The listing builds one solid part. Answer for the finished solid, in the listing's coordinates (mm). Coordinates: 2 decimals unless noted, no trailing zeros. Loops run counter-clockwise (first coordinate to the right, second up) from the corner with the lowest first, then second, coordinate; pieces in that order, holes last. Notation, with made-up numbers: M -5.5,-21.75 L 37.5,-21.75 A14 cw 37.5,-7.75 Z; hole C -14,26 d3. An arc over 180 degrees is marked long. Answer in a Markdown table with one row per item. Add a question column.
from build123d import *

# Parameters (mm, degrees)
SKETCH2_W           = 40
SKETCH2_H           = 80
BOSS_EXTRUDE1_DEPTH = 5
CUT_EXTRUDE1_DEPTH  = 2.8000000000000003
CUT_EXTRUDE2_DEPTH  = 1
CUT_EXTRUDE3_DEPTH  = 1
CUT_EXTRUDE4_DEPTH  = 0.5
CUT_EXTRUDE5_DEPTH  = 0.5
FILLET1_R           = 0.5
FILLET2_R           = 2.5
F_3DSKETCH6_R       = 1.5500000000000003
F_3DSKETCH6_R_2     = 0.8500000000000008
CUT_EXTRUDE6_DEPTH  = 2.1
FILLET3_START       = -10.446006344
FILLET3_DEPTH       = 8.020486493
FILLET3_START_2     = 2.417038032
FILLET3_2_DEPTH     = 8.020486493


with BuildPart() as part:
    # Sketch2 → Boss-Extrude1 (new body)
    with BuildSketch(Plane(origin=(0, 0, 0), x_dir=(1, 0, 0), z_dir=(0, 1, 0))):
        Rectangle(SKETCH2_W, SKETCH2_H)
    extrude(amount=BOSS_EXTRUDE1_DEPTH)

    # 3DSketch1 → Cut-Extrude1 (cut)
    with BuildSketch(Plane(origin=(-16.51128006150057, 0, -37.5), x_dir=(0.4458957716594368, 0, 0.8950848902848463), z_dir=(0, 1, 0))):
        Polygon((0, 0), (14.72461992821574, 29.557994604621218), (74.05892188684597, 0), (59.334301958630235, -29.557994604621218), align=None)
    extrude(amount=CUT_EXTRUDE1_DEPTH, mode=Mode.SUBTRACT)

    # 3DSketch2 → Cut-Extrude2 (cut)
    with BuildSketch(Plane(origin=(2.4170380320342884, 0, 29.789021971701544), x_dir=(-0.7832232950206466, 0, 0.621740516724623), z_dir=(0, 1, 0))):
        Polygon((0, 0), (-6.28183185870911, 4.986661416535171), (0.06674689686894317, 12.984137273242512), (6.348578755578054, 7.997475856707341), align=None)
        Polygon((3.7928041411073767, -3.0108144401721697), (10.074635999816486, -7.997475856707341), (16.42321475539454, 0), (10.14138289668543, 4.986661416535171), align=None)
    extrude(amount=CUT_EXTRUDE2_DEPTH, mode=Mode.SUBTRACT)

    # 3DSketch3 → Cut-Extrude3 (cut)
    with BuildSketch(Plane(origin=(2.4170380320342884, 1, 40), x_dir=(-0.9548954301559858, 0.29694227968953, 0), z_dir=(0, 0, -1))):
        Polygon((0, 0), (-7.658725899785049, 2.3816215434478725), (-6.470956781026929, 6.2012032640718155), (1.1877691187581199, 3.8195817206239426), align=None)
        Polygon((12.282862292108083, -3.8195817206239426), (4.6241363923230345, -1.43796017717607), (5.811905511081154, 2.381621543447873), (13.470631410866202, 0), align=None)
    extrude(amount=CUT_EXTRUDE3_DEPTH, mode=Mode.SUBTRACT)

    # 3DSketch4 → Cut-Extrude4 (cut)
    with BuildSketch(Plane(origin=(-10.446006343517528, 5, 39), x_dir=(0.25565796932804924, 0, -0.9667672950193641), z_dir=(0, 1, 0))):
        Polygon((0, 0), (76.37461630652976, 20.19697957691589), (78.42511759635093, 12.443035545347499), (2.0505012898211623, -7.753944031568391), align=None)
        Polygon((3.288539804430162, -12.435570616666274), (79.66315611095993, 7.761408960249617), (81.71563147305025, 0), (5.341015166520477, -20.19697957691589), align=None)
    extrude(amount=-CUT_EXTRUDE4_DEPTH, mode=Mode.SUBTRACT)

    # 3DSketch5 → Cut-Extrude5 (cut)
    with BuildSketch(Plane(origin=(10.445246061241729, 4.500000000000001, -11.016513850599985), x_dir=(-0.3854175434043051, 0, 0.9227422810493678), z_dir=(0, 1, 0))):
        Polygon((0, 0), (3.0942122165558494, -7.407966989609723), (49.24656429719578, 11.869274908335926), (46.152352080639936, 19.27724189794565), align=None)
        Polygon((23.45245782033335, -4.152597437612319), (26.543694021369404, -11.553439439280611), (54.20420726112153, 0), (51.11297106008547, 7.400842001668292), align=None)
    extrude(amount=-CUT_EXTRUDE5_DEPTH, mode=Mode.SUBTRACT)

    # Fillet1
    fillet1_edges = [part.edges().sort_by_distance(p)[0] for p in [
        (-10.446006343517528, 5, 7.11e-15),
        (2.4170380320342884, 5, 0),
        (10.445246061241729, 5, -0.5000000000000071),
    ]]
    fillet(fillet1_edges, radius=FILLET1_R)

    # Fillet2
    fillet2_edges = [part.edges().sort_by_distance(p)[0] for p in [
        (-20, 5, 0),
        (20, 5, 0),
    ]]
    fillet(fillet2_edges, radius=FILLET2_R)

    # 3DSketch6 → Cut-Extrude6 (cut)
    with BuildSketch(Plane(origin=(15.004520440934186, 0, 34.437112055137284), x_dir=(-0.41484987007197305, 0, -0.909889875370238), z_dir=(0, -1, 0))):
        with Locations(Location((0, 0, 0), (0, 0, 24.509862444))):
            Circle(F_3DSKETCH6_R)
        with Locations(Location((12.4516160827032, -27.310119209349818, 0), (0, 0, 24.509862444))):
            Circle(F_3DSKETCH6_R)
        with Locations(Location((80.16037328194126, 0, 0), (0, 0, 24.509862444))):
            Circle(F_3DSKETCH6_R_2)
        with Locations(Location((65.01761603264471, 33.2125968942302, 0), (0, 0, 24.509862444))):
            Circle(F_3DSKETCH6_R_2)
    extrude(amount=-CUT_EXTRUDE6_DEPTH, mode=Mode.SUBTRACT)

    # Fillet3: read off the stored shape, not the designer's step
    # Fillet3 outline → Fillet3 (cut)
    with BuildSketch(Plane.YZ.offset(FILLET3_START)):
        with BuildLine():
            Line((0, 28.789021972), (0.580987425, 28.789021972))
            ThreePointArc((0.580987425, 28.789021972), (0.776930768, 29.294705016), (1, 29.789021972))
            Line((1, 29.789021972), (0, 29.789021972))
            Line((0, 29.789021972), (0, 28.789021972))
        make_face()
    extrude(amount=FILLET3_DEPTH, mode=Mode.SUBTRACT)

    # Fillet3 2 outline → Fillet3 2 (cut)
    with BuildSketch(Plane.YZ.offset(FILLET3_START_2)):
        with BuildLine():
            Line((0, 28.789021972), (0.580987425, 28.789021972))
            ThreePointArc((0.580987425, 28.789021972), (0.776930768, 29.294705016), (1, 29.789021972))
            Line((1, 29.789021972), (0, 29.789021972))
            Line((0, 29.789021972), (0, 28.789021972))
        make_face()
    extrude(amount=FILLET3_2_DEPTH, mode=Mode.SUBTRACT)


solid = part.part
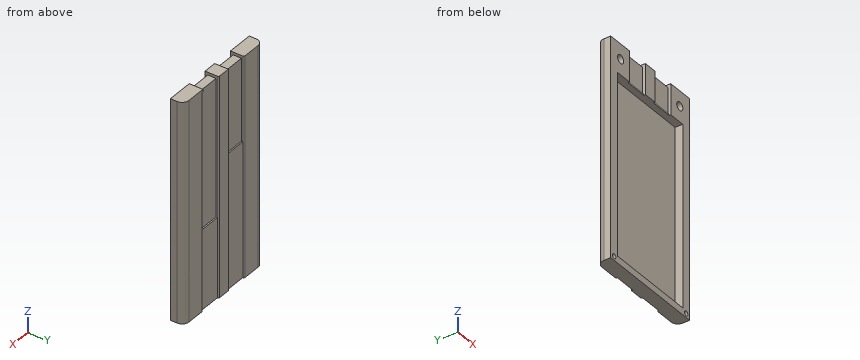
(1) Straight lines are drawn through the part: line 1 (X direction, y = 1.1, z = -38.5); line 2 (Z direction, x = 2, y = 1.1); line 3 (Z direction, x = -9.5, y = 1.15). For each, find the intervals that lie inside material, in ascending order.
(2) A cutting plane is placed at A-A (x = 6.5). Give the vertices of the cut face in (y, z).
(3) Each of these flat-tipped pins is pushed along its axis until it touches: pin 1 (2 mm diameter, centred on x = 2.5, y = 3.5, fed in from +Z); pin 2 (2.5 mm diameter, centred on x = 15, z = 34.44, fed in from -Y); pin 3 (2.5 mm diameter, centred on x = 7, z = 32.5, fed in from -Y); pin 4 (6.5 mm diameter, centred on x = -6, z = 17, fed in from +Y). Where does it stop, or does it pass through?
(4) A cutting plane is placed at D-D (x = -5). Give the vertices of the cut face in (y, z).
(5) A cutting plane is placed at B-B (z = 12). Give the vertices of the cut face in (x, y).
(6) A cutting plane is placed at C-C (z = -38.5). Give the vertices of the cut face in (x, y), plus the area to 3 significant figures.
Solved:
| question | item | result |
|---|---|---|
| 1 | line 1 | x = -20 to -19.1, -17.4 to 17.4, 19.1 to 20 |
| 1 | line 2 | z = -40 to -37.5, 28.79 to 40 |
| 1 | line 3 | z = -40 to -37.5, 28.79 to 39 |
| 2 | outline | M 0,-40 L 4.5,-40 L 4.5,-11.02 L 4,-11.02 L 4,39 L 1,39 L 1,29.79 A10 ccw 0.58,28.79 L 2.8,28.79 L 2.8,-37.5 L 0,-37.5 Z |
| 3 | pin 1 | stops at z = 40 |
| 3 | pin 2 | stops at y = 2.1 |
| 3 | pin 3 | stops at y = 1 |
| 3 | pin 4 | stops at y = 4 |
| 4 | outline | M 0,-40 L 4.5,-40 L 4.5,9.02 L 4,9.02 L 4,39 L 1,39 L 1,29.79 A10 ccw 0.58,28.79 L 2.8,28.79 L 2.8,-37.5 L 0,-37.5 Z |
| 5 | outline | M -20,0 L -16.51,0 L -16.51,2.8 L 16.51,2.8 L 16.51,0 L 20,0 L 20,2.5 A2.5 ccw 17.5,5 L 10.95,5 A0.5 ccw 10.45,4.5 L 10.45,4 L 2.42,4 L 2.42,4.5 A0.5 ccw 1.92,5 L -2.43,5 L -2.43,4 L -10.45,4 L -10.45,4.5 A0.5 ccw -10.95,5 L -17.5,5 A2.5 ccw -20,2.5 Z |
| 6 | outline | M -20,0 L -19.1,0 L -19.1,2.1 L -17.4,2.1 L -17.4,0 L 17.4,0 L 17.4,2.1 L 19.1,2.1 L 19.1,0 L 20,0 L 20,2.5 A2.5 ccw 17.5,5 L 10.95,5 A0.5 ccw 10.45,4.5 L 2.42,4.5 A0.5 ccw 1.92,5 L -2.43,5 L -2.43,4.5 L -10.45,4.5 A0.5 ccw -10.95,5 L -17.5,5 A2.5 ccw -20,2.5 Z |
| 6 | area | 182 mm² |
